```python
from build123d import *
from build123d.topology import SkipClean

# Parameters (mm, degrees)
CROQUIS1_R                   = 2.5
CROQUIS1_R_2                 = 1.5
SALIENTE_EXTRUIR1_DEPTH      = 3
SALIENTE_EXTRUIR2_DEPTH      = 3.078873
SALIENTE_EXTRUIR2_DEPTH_BACK = 2.921127
CROQUIS2_R                   = 2.5
CROQUIS2_R_2                 = 1.5


with BuildPart() as part:
    # Croquis1 → Saliente-Extruir1 (new body)
    # profile 1 of 3: a face of its own
    with BuildSketch(Plane.XY):
        with BuildLine():
            Line((191.551801515, -27.168993214), (169.551801515, -27.168993214))
            ThreePointArc((169.551801515, -27.168993214), (171.319568468, -27.901226261), (172.051801515, -29.668993214))
            ThreePointArc((172.051801515, -29.668993214), (171.319568468, -31.436760167), (169.551801515, -32.168993214))
            Line((169.551801515, -32.168993214), (191.551801515, -32.168993214))
            ThreePointArc((191.551801515, -32.168993214), (189.051801515, -29.668993214), (191.551801515, -27.168993214))
        make_face()
    # profile 2 of 3: a face of its own
    with BuildSketch(Plane.XY):
        with Locations((191.551801515, -29.668993214)):
            Circle(CROQUIS1_R)
        with Locations((191.551801515, -29.668993214)):
            Circle(CROQUIS1_R_2, mode=Mode.SUBTRACT)
    # profile 3 of 3: a face of its own
    with BuildSketch(Plane.XY):
        with Locations((169.551801515, -29.668993214)):
            Circle(CROQUIS1_R)
        with Locations((169.551801515, -29.668993214)):
            Circle(CROQUIS1_R_2, mode=Mode.SUBTRACT)
    extrude(amount=SALIENTE_EXTRUIR1_DEPTH)

    # Croquis2 → Saliente-Extruir2 (add, two sides: drawn at the far end of the back side and taken through both)
    with SkipClean():  # the faces are left unmerged after this step: merging them gives an invalid solid
        with BuildSketch(Plane(origin=(0, 0, 1.5), x_dir=(-1, 0, 0), z_dir=(0, 0, -1)).offset(-SALIENTE_EXTRUIR2_DEPTH_BACK)):
            with Locations(Location((-169.551801515, -29.668993214, 0), (0, 0, 90))):
                Circle(CROQUIS2_R)
            with Locations(Location((-169.551801515, -29.668993214, 0), (0, 0, 286.214321969))):
                Circle(CROQUIS2_R_2, mode=Mode.SUBTRACT)
        extrude(amount=SALIENTE_EXTRUIR2_DEPTH + SALIENTE_EXTRUIR2_DEPTH_BACK)


solid = part.part
```
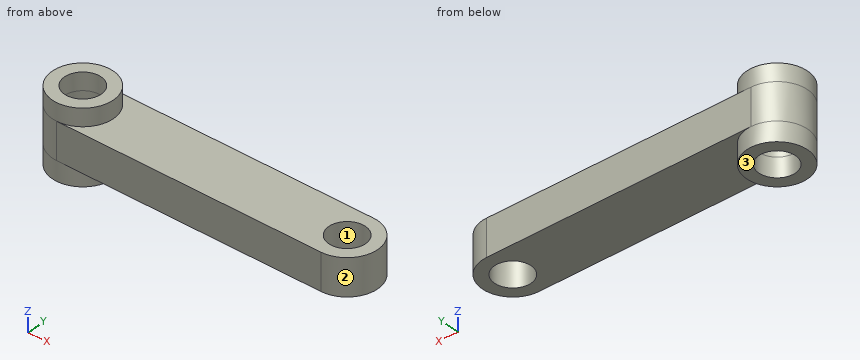
Work out the finished part from the listing and answer in its coordinate system (mm). Face numbers are marked on the shaded views. Coordinates: 2 decimals unless noted, no trailing zeros. Loops run counter-clockwise (first coordinate to the right, second up) from the corner with the lowest first, then second, coordinate; pieces in that order, holes last. Notation, with made-up numbers: (-13.75, 82.5) - (24.25, 82.5) arc R28 cw to (24.25, 119.5) - close; hole circle Ø4 at (66.5, -8.75). An arc over 180 degrees is marked (long way). Use a Markdown table: item, result.
Item 1: The mould has two halves that part along X. Classify the marked faces 1, 2 and 3: +X half, -X half, draft (parallel to the pull), parting line (faces both ways), or undercut.
Evaluation:
| item | result |
|---|---|
| face 1 | undercut |
| face 2 | +X half |
| face 3 | draft |
Item 2: Find section D-D, the plane y = -27.55. Determine the outline of the cut face in (x, z).
Evaluation:
| item | result |
|---|---|
| outline | (168.23, -1.58) - (170.88, -1.58) - (170.88, 0) - (192.88, 0) - (192.88, 3) - (170.88, 3) - (170.88, 4.42) - (168.23, 4.42) - close |
Item 3: Consider probe 1 along Y at (x, z) = (169.5, 3.1); probe 2 along X at (y, z) = (-29.6, -0.25); probe 3 along X at (y, z) = (-29.4, 0.55). Determine where each line is inside the solid, lowest interval first. Write a range as from..to.
Evaluation:
| item | result |
|---|---|
| probe 1 | y = -32.17..-31.17, -28.17..-27.17 |
| probe 2 | x = 167.05..168.05, 171.05..172.05 |
| probe 3 | x = 167.07..168.08, 171.03..190.08, 193.03..194.04 |
Item 4: Find section C-C, the plane z = -1.2. Determine the outline of the cut face in (x, y).
Evaluation:
| item | result |
|---|---|
| outline | circle Ø5 at (169.55, -29.67); hole circle Ø3 at (169.55, -29.67) |
Item 5: Find section B-B, the plane y = -29.05. Determine the outline of the cut face in (x, z), and give its area (3 significant figures).
Evaluation:
| item | result |
|---|---|
| outline | (167.13, -1.58) - (168.19, -1.58) - (168.19, 4.42) - (167.13, 4.42) - close; (170.92, -1.58) - (171.97, -1.58) - (171.97, 0) - (190.19, 0) - (190.19, 3) - (171.97, 3) - (171.97, 4.42) - (170.92, 4.42) - close; (192.92, 0) - (193.97, 0) - (193.97, 3) - (192.92, 3) - close |
| area | 70.5 mm2 |
Item 6: Given pin 1 Ø2.5 at (x, y) = (169.55, -29.67) entering from -Z; pin 2 Ø2.5 at (x, y) = (180.5, -28.5) entering from -Z; pin 3 Ø2.5 at (x, y) = (187.5, -29.5) entering from +Z, each flat-ended and moving along its own axis, determine where each tip first touches the part or whether it passes through.
Evaluation:
| item | result |
|---|---|
| pin 1 | passes through |
| pin 2 | stops at z = 0 |
| pin 3 | stops at z = 3 |
Item 7: Find section A-A, the plane x = 192.25. Determine the outline of the cut face in (y, z), and give its area (3 significant figures).
Evaluation:
| item | result |
|---|---|
| outline | (-32.07, 0) - (-31, 0) - (-31, 3) - (-32.07, 3) - close; (-28.34, 0) - (-27.27, 0) - (-27.27, 3) - (-28.34, 3) - close |
| area | 6.44 mm2 |
